Answer from the drawing. Dimensions are ordinates in mm from the lowest x, y and z of the part. A direction names the side the tool comes from. Round coordinates to 2 decimals unless told otherwise and drop trailing zeros. Write each loop counter-clockwise with the first axis right and the second up, starting at its lowest first coordinate (ties: lowest second). Pieces come first, ordered by that corner, then holes. Notation, with made-up numbers: (25.25, -26) - (68.25, -26) arc R27 ccw to (68.25, 13) - close; hole circle Ø5 at (63, 71). An arc over 180 degrees is marked (long way). Use a Markdown table: item, result. Add a question column.
1) Determine the mould class of the marked faces 4, 5 and 6 for opening direction X: +X half, -X half, draft (parallel to the pull), parting line (faces both ways), or undercut.
2) A cutting plane is placed at D-D (y = 13.5). Give the vertices of the cut face in (x, z), then the cut area to 3 significant figures.
3) A cutting plane is placed at A-A (y = 47.5). Give the vertices of the cut face in (x, z) (1 decimal).
4) Each of these flat-tipped pins is pushed along its axis until it touches: P1, Ø4, axis at x = 24, y = 8.5, coming from the +Z side (1 decimal); P2, Ø2, axis at y = 60, z = 69, coming from the -X side; P3, Ø6, axis at y = 14, z = 57.5, coming from the -X side. Where does it stop, or does it pass through?
5) A tool of negligible diameter and unlimited length cuts with its end or side. For the marked faces 1, 2 and 3, from which of +Z, -Z, +X, -X, +Y, -Y can it reach the whole face along a straight path? Write none if from no direction.
6) Find the intervals of material crossed by probe 1 along X at (y, z) = (59, 73.5); probe 2 along Y at (x, z) = (50, 30); probe 3 along Y at (x, z) = (25.5, 97.5), in increasing order. Write a range as from..to.
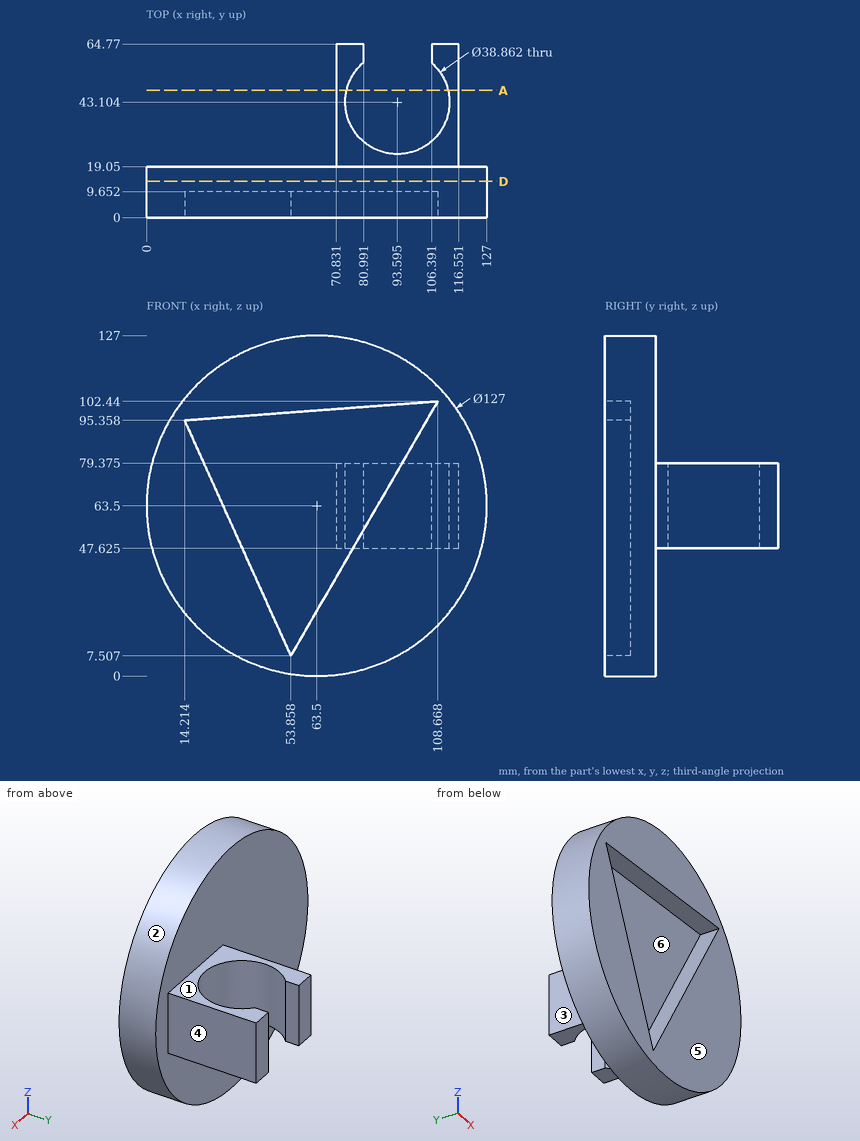
Entries:
| question | item | result |
|---|---|---|
| 1 | face 4 | +X half |
| 1 | face 5 | draft |
| 1 | face 6 | undercut |
| 2 | outline | circle Ø127 at (63.5, 63.5) |
| 2 | area | 12,700 mm² |
| 3 | outline | (70.8, 47.6) - (74.7, 47.6) - (74.7, 79.4) - (70.8, 79.4) - close; (112.5, 47.6) - (116.6, 47.6) - (116.6, 79.4) - (112.5, 79.4) - close |
| 4 | P1 | stops at z = 114.7 |
| 4 | P2 | stops at x = 70.83 |
| 4 | P3 | stops at x = 0.07 |
| 5 | face 1 | +Z, +X, -X, +Y |
| 5 | face 2 | +Y, -Y |
| 5 | face 3 | +Z, -Z, -X, +Y |
| 6 | probe 1 | x = 70.83..80.99, 106.39..116.55 |
| 6 | probe 2 | y = 9.65..19.05 |
| 6 | probe 3 | y = 0..19.05 |
